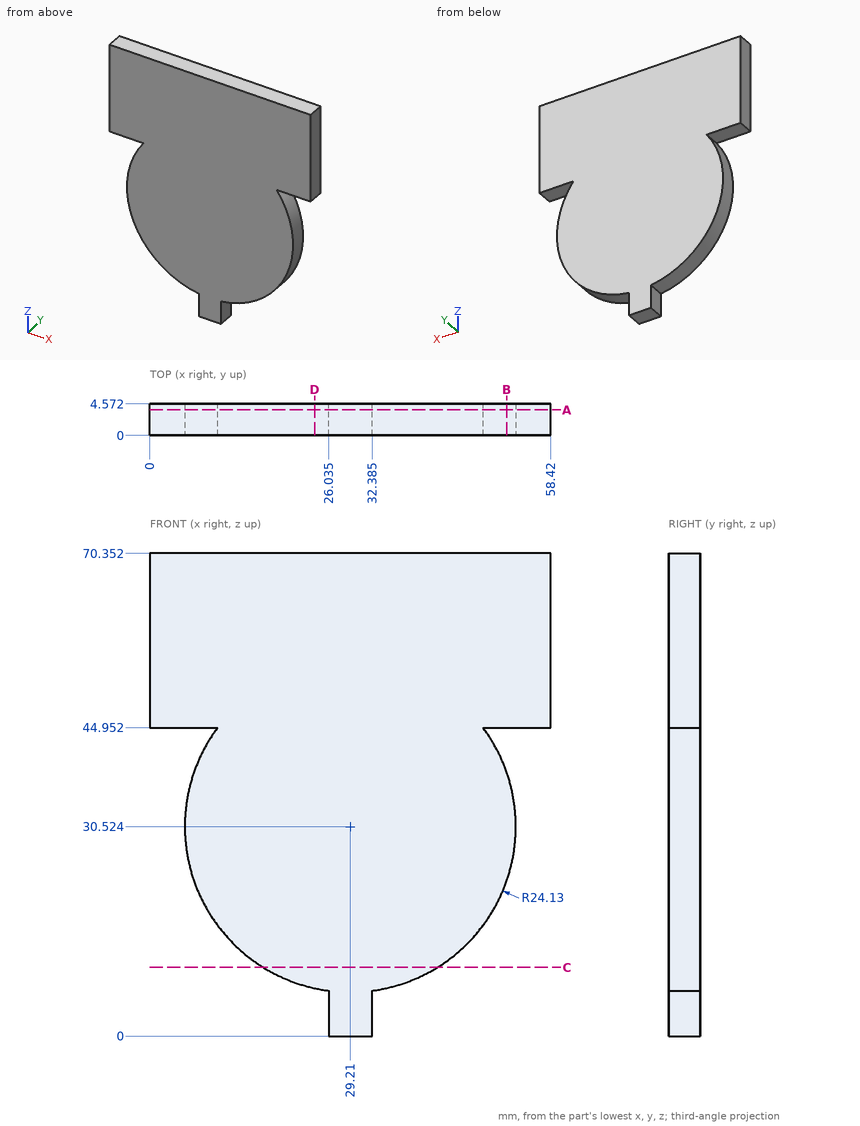
Source: three-view drawing plus pictorial views. Frame: mm from the lowest corner of the part. Coordinates: 2 decimals unless noted, no trailing zeros. Write each loop counter-clockwise with the first axis right and the second up, starting at its lowest first coordinate (ties: lowest second). Pieces come first, ordered by that corner, then holes. Notation, with made-up numbers: (61, 62) - (84, 62) arc R28 cw to (84, 85) - close; hole circle Ø7 at (-10.75, -19). An arc over 180 degrees is marked (long way). Return JSON: item names as keys, results as strings.
Item 1: Section query D-D (x = 24). Output: boundary loops of the cut face in (y, z).
Completed:
{"outline": "(0, 6.96) - (4.57, 6.96) - (4.57, 70.35) - (0, 70.35) - close"}
Item 2: Pin query (flat end, axial travel): pin 1 Ø1 at (y, z) = (1.5, 41) entering from -X; pin 2 Ø1.4 at (x, y) = (6.5, 2.5) entering from -Z (1 decimal); pin 3 Ø1.4 at (y, z) = (2.5, 4) entering from +X (3 decimals). Return the tip coordinate at first contact, or that it passes through.
Completed:
{"pin 1": "stops at x = 7.24", "pin 2": "stops at z = 20.6", "pin 3": "stops at x = 32.385"}
Item 3: Section query A-A (y = 3.7). Output: boundary loops of the cut face in (x, z) (1 decimal).
Completed:
{"outline": "(0, 45) - (9.9, 45) arc R24.1 ccw to (26, 6.6) - (26, 0) - (32.4, 0) - (32.4, 6.6) arc R24.1 ccw to (48.6, 45) - (58.4, 45) - (58.4, 70.4) - (0, 70.4) - close"}
Item 4: Line query: L1, parallel to X at y = 2.1, z = 21; L2, parallel to X at y = 4.2, z = 22.5; L3, parallel to Z at x = 54, y = 1.4. Output: solid intervals per line, ascending.
Completed:
{"L1": "x = 7.04 to 51.38", "L2": "x = 6.45 to 51.97", "L3": "z = 44.95 to 70.35"}
Item 5: Section query C-C (z = 10). Output: boundary loops of the cut face in (x, y).
Completed:
{"outline": "(16.52, 0) - (41.9, 0) - (41.9, 4.57) - (16.52, 4.57) - close"}
Item 6: Section query B-B (x = 52). Output: boundary loops of the cut face in (y, z) (1 decimal).
Completed:
{"outline": "(0, 22.6) - (4.6, 22.6) - (4.6, 38.5) - (0, 38.5) - close; (0, 45) - (4.6, 45) - (4.6, 70.4) - (0, 70.4) - close"}
